Read the model definition and answer for the solid it produces. Units are mm, in the model's axes. Face numbers are marked on the shaded views. A direction names the side the tool comes from. Give positions to 0.01 mm unless a question says otherwise; leave off trailing zeros. Order: outer loops, then holes, each group sorted by start corner. A loop starts at its lowest first (then second) coordinate and runs counter-clockwise, first axis right, second up. Notation, with made-up numbers: (16.25, 18.5) - (51.25, 18.5) arc R5 cw to (51.25, 25.5) - close; hole circle Ø11 at (12.25, 68). An arc over 180 degrees is marked (long way). Use a Markdown table: item, result. Add a question column.
1. A cutting plane is placed at C-C on x = 28.2. Determine the outline of the cut face in (y, z), and give its area (3 significant figures).
2. A cutting plane is placed at B-B on y = 28.2. Determine the outline of the cut face in (x, z), and give its area (3 significant figures).
3. A cutting plane is placed at A-A on z = 97.5. Determine the outline of the cut face in (x, y).
4. Consider L1, parallel to Y at x = 4.63, z = 97.1; L2, parallel to Y at x = 4, z = 96; L3, parallel to Z at x = 22, y = 36. Determine where each line is inside the solid, lowest interval first.
5. Flat-ended cylindrical pins translate along their axes: P1, Ø2, axis at y = 54.5, z = 42, coming from the -X side; P2, Ø8, axis at x = 15.5, z = 110.5, coming from the -Y side; P3, Ø3, axis at y = 1.5, z = 24, coming from the +X side; P4, Ø7, axis at x = 27.5, z = 111.5, coming from the +Y side. Find the tip coordinate at first contact, or state that the pin passes through.
6. A cutting plane is placed at D-D on y = 46. Determine the outline of the cut face in (x, z), and give its area (3 significant figures).
7. Which of the six approach directions +Z, -Z, +X, -X, +Y, -Y give full straight-line access (tool end or side, diameter ignored) to the marked faces 1 and 2?
```python
from build123d import *

# Parameters (mm, degrees)
SKETCH_1_W          = 56.4
SKETCH_1_H          = 56.4
EXTRUDE_1_DEPTH     = 99.5
SKETCH_2_R          = 19.05
EXTRUDE_2_DEPTH     = 1.6
SKETCH_3_R          = 5
EXTRUDE_3_DEPTH     = 25
SKETCH_4_W          = 8.660254038
SKETCH_4_H          = 6.0292226
CUT_EXTRUDE_1_DEPTH = 20
CUT_EXTRUDE_2_DEPTH = 94.8
SKETCH_6_R          = 2.5
CUT_EXTRUDE_3_DEPTH = 94.8
FILLET_1_R          = 5


with BuildPart() as part:
    # 草图1 → 凸台-拉伸1 (new body)
    with BuildSketch(Plane.XY):
        with Locations((28.2, 28.2)):
            Rectangle(SKETCH_1_W, SKETCH_1_H)
    extrude(amount=EXTRUDE_1_DEPTH)

    # 草图2 → 凸台-拉伸2 (add)
    with BuildSketch(Plane.XY.offset(99.5)):
        with Locations((28.2, 28.2)):
            Circle(SKETCH_2_R)
    extrude(amount=EXTRUDE_2_DEPTH)

    # 草图3 → 凸台-拉伸3 (add)
    with BuildSketch(Plane.XY.offset(101.1)):
        with Locations((28.2, 28.2)):
            Circle(SKETCH_3_R)
    extrude(amount=EXTRUDE_3_DEPTH)

    # 草图4 → 切除-拉伸1 (cut)
    with BuildSketch(Plane.XY.offset(126.1)):
        with Locations((28.2, 33.7146113)):
            Rectangle(SKETCH_4_W, SKETCH_4_H)
    extrude(amount=-CUT_EXTRUDE_1_DEPTH, mode=Mode.SUBTRACT)

    # 草图5 → 切除-拉伸2 (cut)
    with BuildSketch(Plane(origin=(0, 0, 0), x_dir=(-1, 0, 0), z_dir=(0, 0, -1))):
        with BuildLine():
            Line((-61.988810655, 58.062513104), (-46.510137618, 58.062513104))
            Line((-46.510137618, 58.062513104), (-46.510137618, 52.340700561))
            ThreePointArc((-46.510137618, 52.340700561), (-47.974603712, 48.805166655), (-51.510137618, 47.340700561))
            Line((-51.510137618, 47.340700561), (-61.988810655, 47.340700561))
            Line((-61.988810655, 47.340700561), (-61.988810655, 58.062513104))
        make_face()
        with BuildLine():
            Line((-9.889862382, 58.062513104), (-9.889862382, 52.340700561))
            ThreePointArc((-9.889862382, 52.340700561), (-8.425396288, 48.805166655), (-4.889862382, 47.340700561))
            Line((-4.889862382, 47.340700561), (5.588810655, 47.340700561))
            Line((5.588810655, 47.340700561), (5.588810655, 58.062513104))
            Line((5.588810655, 58.062513104), (-9.889862382, 58.062513104))
        make_face()
        with BuildLine():
            Line((5.588810655, -1.662513104), (-9.889862382, -1.662513104))
            Line((-9.889862382, -1.662513104), (-9.889862382, 4.059299439))
            ThreePointArc((-9.889862382, 4.059299439), (-8.425396288, 7.594833345), (-4.889862382, 9.059299439))
            Line((-4.889862382, 9.059299439), (5.588810655, 9.059299439))
            Line((5.588810655, 9.059299439), (5.588810655, -1.662513104))
        make_face()
        with BuildLine():
            Line((-46.510137618, -1.662513104), (-46.510137618, 4.059299439))
            ThreePointArc((-46.510137618, 4.059299439), (-47.974603712, 7.594833345), (-51.510137618, 9.059299439))
            Line((-51.510137618, 9.059299439), (-61.988810655, 9.059299439))
            Line((-61.988810655, 9.059299439), (-61.988810655, -1.662513104))
            Line((-61.988810655, -1.662513104), (-46.510137618, -1.662513104))
        make_face()
    extrude(amount=-CUT_EXTRUDE_2_DEPTH, mode=Mode.SUBTRACT)

    # 草图6 → 切除-拉伸3 (cut)
    with BuildSketch(Plane.XY.offset(99.5)):
        with Locations((4.63, 51.77)):
            Circle(SKETCH_6_R)
        with Locations((51.77, 51.77)):
            Circle(SKETCH_6_R)
        with Locations((51.77, 4.63)):
            Circle(SKETCH_6_R)
        with Locations((4.63, 4.63)):
            Circle(SKETCH_6_R)
    extrude(amount=-CUT_EXTRUDE_3_DEPTH, mode=Mode.SUBTRACT)

    # 圆角1
    fillet_1_edges = [part.edges().sort_by_distance(p)[0] for p in [
        (0, 56.4, 97.15),
        (56.4, 56.4, 97.15),
        (56.4, 0, 97.15),
        (0, 0, 97.15),
    ]]
    fillet(fillet_1_edges, radius=FILLET_1_R)


solid = part.part
```
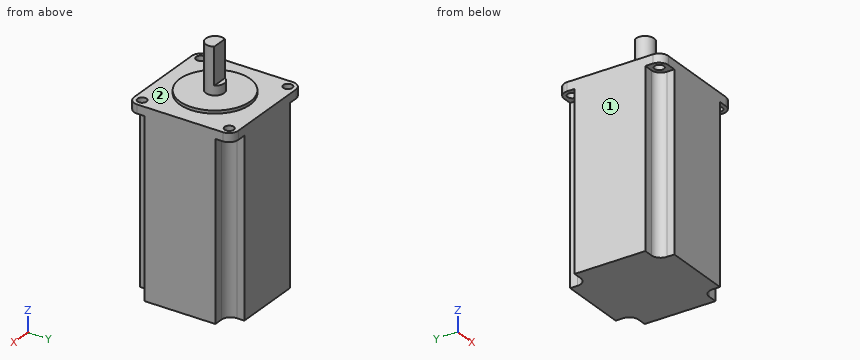
Output values:
| question | item | result |
|---|---|---|
| 1 | outline | (0, 0) - (56.4, 0) - (56.4, 99.5) - (47.25, 99.5) - (47.25, 101.1) - (33.2, 101.1) - (33.2, 106.1) - (30.7, 106.1) - (30.7, 126.1) - (23.2, 126.1) - (23.2, 101.1) - (9.15, 101.1) - (9.15, 99.5) - (0, 99.5) - close |
| 1 | area | 5,870 mm² |
| 2 | outline | (0, 0) - (56.4, 0) - (56.4, 99.5) - (47.25, 99.5) - (47.25, 101.1) - (33.2, 101.1) - (33.2, 126.1) - (23.2, 126.1) - (23.2, 101.1) - (9.15, 101.1) - (9.15, 99.5) - (0, 99.5) - close |
| 2 | area | 5,920 mm² |
| 3 | outline | (0, 5) arc R5 ccw to (5, 0) - (51.4, 0) arc R5 ccw to (56.4, 5) - (56.4, 51.4) arc R5 ccw to (51.4, 56.4) - (5, 56.4) arc R5 ccw to (0, 51.4) - close; hole circle Ø5 at (4.63, 4.63); hole circle Ø5 at (4.63, 51.77); hole circle Ø5 at (51.77, 4.63); hole circle Ø5 at (51.77, 51.77) |
| 4 | L1 | 0.01 to 2.13, 7.13 to 49.27, 54.27 to 56.39 |
| 4 | L2 | 0.1 to 2.21, 7.05 to 49.35, 54.19 to 56.3 |
| 4 | L3 | 0 to 101.1 |
| 5 | P1 | x = 9.89 |
| 5 | P2 | through |
| 5 | P3 | x = 46.51 |
| 5 | P4 | y = 30.7 |
| 6 | outline | (0, 0) - (56.4, 0) - (56.4, 99.5) - (34.99, 99.5) - (34.99, 101.1) - (21.41, 101.1) - (21.41, 99.5) - (0, 99.5) - close |
| 6 | area | 5,630 mm² |
| 7 | face 1 | +Z, -Z, -X, +Y, -Y |
| 7 | face 2 | +Z |
